Geometry check sheet. Reference: the model listing, model coordinates, mm. Round coordinates to 2 decimals unless told otherwise and drop trailing zeros. Order: outer loops, then holes, each group sorted by start corner. A loop starts at its lowest first (then second) coordinate and runs counter-clockwise, first axis right, second up.
(1) Material ranges on line 1 along Z through (x, y) = (6, 0.35); line 2 along X through (y, z) = (0.55, -6.75); line 3 along Y through (x, z) = (17.25, -0.5), recorded low to high.
(2) Sectioned sample at A-A (y = 0.4). Record the boundary of the cut face in (x, z).
(3) Sectioned sample at B-B (x = 16). Record the boundary of the cut face in (y, z), plus the area to 3 significant figures.
Autodesk Inventor part; units mm, degrees
ref_plane "YZ Plane" through (0, 0, 0) normal (1, 0, 0) x (0, 1, 0)
ref_plane "XZ Plane" through (0, 0, 0) normal (0, 1, 0) x (-1, 0, 0)
ref_plane "XY Plane" through (0, 0, 0) normal (0, 0, 1) x (1, 0, 0)
sketch "Sketch1" plane through (0, 0, 0) normal (0, 1, 0) x (-1, 0, 0)
  line L0 (0, 0) -> (-29, 0)
  line L1 (-29, 0) -> (-29, -9.5)
  line L2 (-29, -9.5) -> (0, -9.5)
  line L3 (0, -9.5) -> (0, 0)
  dimension "d0" = 29
  dimension "d1" = 9.5
extrude "Extrusion1" add sketch "Sketch1" along normal blind 4.3
fillet "Fillet1" radius 1 12 edges at (0, 0, -4.75) (0, 2.15, 0) (0, 4.3, -4.75) (0, 2.15, -9.5) (14.5, 0, -9.5) (14.5, 4.3, -9.5) (29, 2.15, -9.5) (29, 0, -4.75) (29, 4.3, -4.75) (29, 2.15, 0) (14.5, 0, 0) (14.5, 4.3, 0)
properties part number "Magnet3010" material "Stainless Steel"
Answer below:
1. line 1: z = -9.26 to -0.24
1. line 2: x = 0.11 to 28.89
1. line 3: y = 0.13 to 4.17
2. outline: (0.2, -8.5) arc R0.8 ccw to (1, -9.3) - (28, -9.3) arc R0.8 ccw to (28.8, -8.5) - (28.8, -1) arc R0.8 ccw to (28, -0.2) - (1, -0.2) arc R0.8 ccw to (0.2, -1) - close
3. outline: (0, -8.5) arc R1 ccw to (1, -9.5) - (3.3, -9.5) arc R1 ccw to (4.3, -8.5) - (4.3, -1) arc R1 ccw to (3.3, 0) - (1, 0) arc R1 ccw to (0, -1) - close
3. area: 40.0 mm2
